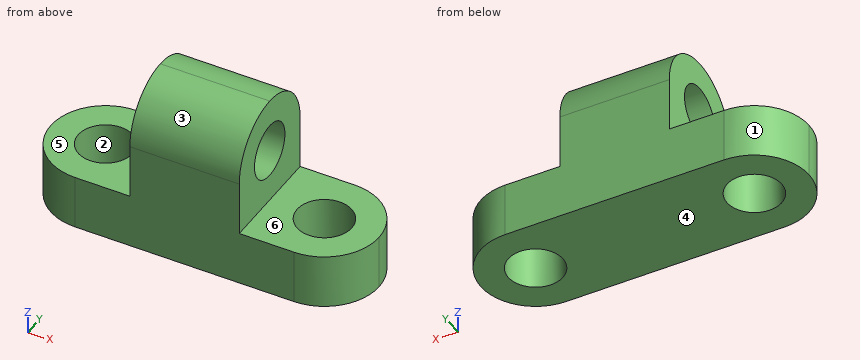
from build123d import *

# Parameters (mm, degrees)
F1_DEPTH  = 25.4
F2_R      = 12.7
F3_R      = 12.69999
F4_R      = 12.7
F5_R      = 12.69999
F6_R      = 12.7
F7_R      = 12.69999
F8_R      = 6.35
F9_DEPTH  = 25.4
F10_R     = 6.35
F11_DEPTH = 25.4
F12_R     = 6.35
F13_DEPTH = 25.4


# Not quite as in the source:
# - a fillet or chamfer is up to 0.001 mm smaller than in the source, because OpenCascade refuses the exact size


with BuildPart() as f1:
    # F0 (on Front) → F1 (new body)
    with BuildSketch(Plane.XZ):
        Polygon((0, 12.7), (0, 0), (76.2, 0), (76.2, 12.7), (50.8, 12.7), (50.8, 38.1), (25.4, 38.1), (25.4, 12.7), align=None)
    extrude(amount=F1_DEPTH)

    # F2
    f2_edges = [f1.edges().sort_by_distance(p)[0] for p in [
        (76.2, -25.4, 6.35),
    ]]
    fillet(f2_edges, radius=F2_R)

    # F3 (radius 12.7 in the source; OpenCascade refuses exactly that, so slightly less here)
    f3_edges = [f1.edges().sort_by_distance(p)[0] for p in [
        (76.2, 0, 6.35),
    ]]
    fillet(f3_edges, radius=F3_R)

    # F4
    f4_edges = [f1.edges().sort_by_distance(p)[0] for p in [
        (0, -25.4, 6.35),
    ]]
    fillet(f4_edges, radius=F4_R)

    # F5 (radius 12.7 in the source; OpenCascade refuses exactly that, so slightly less here)
    f5_edges = [f1.edges().sort_by_distance(p)[0] for p in [
        (0, 0, 6.35),
    ]]
    fillet(f5_edges, radius=F5_R)

    # F6
    f6_edges = [f1.edges().sort_by_distance(p)[0] for p in [
        (38.1, 0, 38.1),
    ]]
    fillet(f6_edges, radius=F6_R)

    # F7 (radius 12.7 in the source; OpenCascade refuses exactly that, so slightly less here)
    f7_edges = [f1.edges().sort_by_distance(p)[0] for p in [
        (38.1, -25.4, 38.1),
    ]]
    fillet(f7_edges, radius=F7_R)

    # F8 (on face) → F9 (cut)
    with BuildSketch(Plane.YZ.offset(50.8)):
        with Locations((-12.7, 25.4)):
            Circle(F8_R)
    extrude(amount=-F9_DEPTH, mode=Mode.SUBTRACT)

    # F10 (on face) → F11 (cut)
    with BuildSketch(Plane.XY.offset(12.7)):
        with Locations((63.5, -12.7)):
            Circle(F10_R)
    extrude(amount=-F11_DEPTH, mode=Mode.SUBTRACT)

    # F12 (on face) → F13 (cut)
    with BuildSketch(Plane.XY.offset(12.7)):
        with Locations((12.7, -12.7)):
            Circle(F12_R)
    extrude(amount=-F13_DEPTH, mode=Mode.SUBTRACT)


solid = f1.part
Input: part model. Units: mm. Frame: model coordinates. Face numbers are marked on the shaded views. A direction names the side the tool comes from. Give positions to 0.01 mm unless a question says otherwise; leave off trailing zeros. Order: outer loops, then holes, each group sorted by start corner. A loop starts at its lowest first (then second) coordinate and runs counter-clockwise, first axis right, second up. Notation, with made-up numbers: (62, 4) -> (97, 4) arc R20 cw to (97, 28) -> close; hole circle Ø3 at (-15, -28). An arc over 180 degrees is marked (long way). Use one line per item in the form item = value.
1) Reachability of the marked faces 4, 5 and 6 from +Z, -Z, +X, -X, +Y, -Y: full face, straight path, thin tool, end or side. Return the list, or none.
Response values:
face_4 = -Z, +X, -X, +Y, -Y
face_5 = +Z, -X, +Y, -Y
face_6 = +Z, +X, +Y, -Y
2) Section B-B, the plane z = 3. Count the separate pieces of the cut face and the enclosed holes in it, and give its area (3 significant figures).
Response values:
separate_pieces = 1
enclosed_holes = 2
area = 1,540 mm^2
3) First-contact query: pin 1 Ø3 at (y, z) = (-20.5, 7.5) entering from +X; pin 2 Ø10 at (y, z) = (-17.5, 32) entering from +X; pin 3 Ø5 at (x, y) = (32.5, -13) entering from +Z; pin 4 Ø1 at (y, z) = (-5.5, 10) entering from +X. Flat tips, straight axial feed; report the tip coordinate or a pass-through.
Response values:
pin_1 = 74.53
pin_2 = 50.8
pin_3 = 38.1
pin_4 = 74.29
4) Line query: probe 1 along X at (y, z) = (-16, 9); probe 2 along X at (y, z) = (-7.5, 2); probe 3 along Y at (x, z) = (12.7, 3.5). Output: solid intervals per line, ascending.
Response values:
probe_1 = 0.44 to 7.27, 18.13 to 58.07, 68.93 to 75.76
probe_2 = 1.11 to 9.06, 16.34 to 59.86, 67.14 to 75.09
probe_3 = -25.4 to -19.05, -6.35 to 0
5) Mould query, pull axis X, two halves, no side actions, for the marked faces 1, 2 and 3. Classes: pulls with the +X half, pulls with the -X half, needs draft (parallel to the pull), parting line crosses it, or undercut.
Response values:
face_1 = pulls with the -X half
face_2 = undercut
face_3 = needs draft
6) Section C-C, the plane z = 30. Return loops of the section in (x, y).
Response values:
outline = (25.4, -24.54) -> (50.8, -24.54) -> (50.8, -17.08) -> (25.4, -17.08) -> close; (25.4, -8.32) -> (50.8, -8.32) -> (50.8, -0.86) -> (25.4, -0.86) -> close
7) Section D-D, the plane y = -18. Return loops of the section in (x, z).
Response values:
outline = (1.16, 0) -> (9.2, 0) -> (9.2, 12.7) -> (1.16, 12.7) -> close; (16.2, 0) -> (60, 0) -> (60, 12.7) -> (50.8, 12.7) -> (50.8, 21.9) -> (25.4, 21.9) -> (25.4, 12.7) -> (16.2, 12.7) -> close; (25.4, 28.9) -> (50.8, 28.9) -> (50.8, 36.94) -> (25.4, 36.94) -> close; (67, 0) -> (75.04, 0) -> (75.04, 12.7) -> (67, 12.7) -> close
